Autodesk Inventor part; units mm, degrees
ref_plane "Work Plane1" through (0, 0, 400) normal (0, 0, 1) x (1, 0, 0)
ref_plane "Work Plane2" through (0, 0, 100) normal (0, 0, -1) x (-1, 0, 0)
ref_plane "YZ Plane" through (0, 0, 0) normal (1, 0, 0) x (0, 1, 0)
sketch "Sketch1" plane through (0, 0, 0) normal (0, 0, 1) x (1, 0, 0)
  line L0 (-7.5, 3.5) -> (7.5, 3.5)
  line L1 (7.5, 3.5) -> (7.5, -3.5)
  line L2 (7.5, -3.5) -> (-7.5, -3.5)
  line L3 (-7.5, -3.5) -> (-7.5, 3.5)
  line L4 (-7.5, 3.5) -> (7.5, -3.5) construction
  line L5 (7.5, 3.5) -> (-7.5, -3.5) construction
  line L6 (-12.5, 8.5) -> (12.5, 8.5)
  line L7 (12.5, 8.5) -> (12.5, -8.5)
  line L8 (12.5, -8.5) -> (-12.5, -8.5)
  line L9 (-12.5, -8.5) -> (-12.5, 8.5)
  line L10 (-12.5, 8.5) -> (12.5, -8.5) construction
  line L11 (12.5, 8.5) -> (-12.5, -8.5) construction
  line L12 (-7.5, 8.5) -> (-7.5, -8.5)
  point P0 (0, 0)
  dimension "d0" = 15
  dimension "d1" = 7
  dimension "d2" = 25
  dimension "d3" = 17
extrude "Extrusion1" add sketch "Sketch1" along normal blind 500 contours L12 L6 L7 L8 L2 L1 L0
ref_plane "Work Plane1" through (0, 0, 400) normal (0, 0, 1) x (1, 0, 0)
sketch "Sketch2" plane through (0, 0, 400) normal (0, 0, 1) x (1, 0, 0)
  line L0 (-27.5, 8.5) -> (52.5, 8.5)
  line L1 (52.5, 8.5) -> (52.5, -8.5)
  line L2 (52.5, -8.5) -> (-27.5, -8.5)
  line L3 (-27.5, -8.5) -> (-27.5, 8.5)
  line L4 (12.5, -8.5) -> (12.5, 8.5)
  line L5 (-27.5, 8.5) -> (52.5, -8.5) construction
  line L6 (52.5, 8.5) -> (-27.5, -8.5) construction
  line L7 (12.5, 0) -> (52.5, 0)
  line L8 (52.5, 0) -> (52.5, 8.5)
  line L9 (52.5, 8.5) -> (12.5, 8.5)
  line L10 (12.5, 8.5) -> (12.5, 0)
  point P0 (0, 0)
  point P1 (12.5, -6.5)
  point P2 (12.5, 6.5)
  point P3 (12.5, 6.5)
  dimension "d8" = 80
  dimension "d9" = 17
extrude "Extrusion2" add sketch "Sketch2" against normal blind 25 contours L0 L1 L7 L4
ref_plane "Work Plane2" through (0, 0, 100) normal (0, 0, -1) x (-1, 0, 0)
sketch "Sketch3" plane through (0, 0, 100) normal (0, 0, -1) x (-1, 0, 0)
  line L0 (-12.5, 8.5) -> (-12.5, 0)
  line L1 (-12.5, 8.5) -> (-52.5, 8.5)
  line L2 (-52.5, 8.5) -> (-52.5, 0)
  line L3 (-52.5, 0) -> (-12.5, 0)
  point P0 (0, 0)
extrude "Extrusion3" add sketch "Sketch3" against normal blind 25
fillet "Fillet2" radius 7 6 edges at (12.5, 4.25, 100) (12.5, 0, 112.5) (12.5, 4.25, 125) (12.5, 4.25, 375) (12.5, 0, 387.5) (12.5, 4.25, 400)
properties part number "GUIA DE TAPA PRINCIPAL"
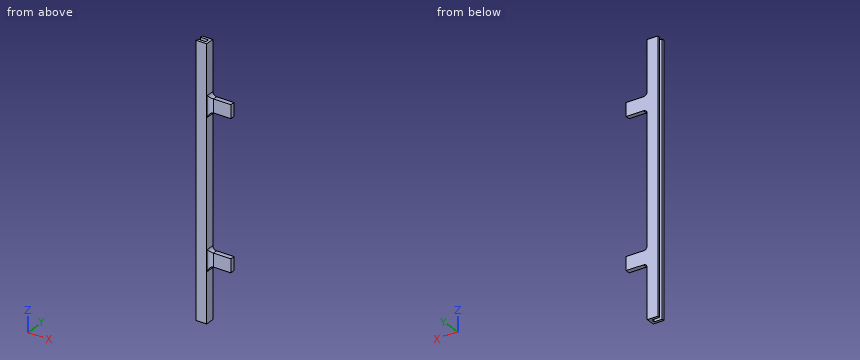
Build history of the part. All positions in model axes, mm. Round coordinates to 2 decimals unless told otherwise and drop trailing zeros. Write each loop counter-clockwise with the first axis right and the second up, starting at its lowest first coordinate (ties: lowest second). Pieces come first, ordered by that corner, then holes. Notation, with made-up numbers: (-32, -7) - (-8, -7) arc R13 ccw to (-8, 5) - close; hole circle Ø9 at (62, 64.25). An arc over 180 degrees is marked (long way). One line per question, with ' | ' between items.
1. Band-saw the part on A-A, the plane x = 1. Write the cut outline in (y, z), and give its area (3 significant figures).
Results are:
outline: (-8.5, 0) - (-3.5, 0) - (-3.5, 500) - (-8.5, 500) - close; (3.5, 0) - (8.5, 0) - (8.5, 500) - (3.5, 500) - close | area: 5,000 mm^2
2. Band-saw the part on C-C, the plane x = 34. Write the cut outline in (y, z).
Results are:
outline: (0, 100) - (8.5, 100) - (8.5, 125) - (0, 125) - close; (0, 375) - (8.5, 375) - (8.5, 400) - (0, 400) - close
3. Drop flat-ended pins along their axis: pin 1 Ø12.5 at (x, z) = (42, 114.5) entering from -Y; pin 2 Ø3.5 at (y, z) = (-0.5, 275.5) entering from -X; pin 3 Ø7 at (x, y) = (33.5, 3) entering from -Z; pin 4 Ø2 at (x, y) = (46.5, -2.5) entering from -Z. Give the stop position or say it passes through.
Results are:
pin 1: y = 0 | pin 2: x = 7.5 | pin 3: z = 100 | pin 4: through
4. Drill centre lines: line 1 along Y through (x, z) = (-0.5, 72); line 2 along Z through (x, y) = (40, 3.25); line 3 along X through (y, z) = (7.25, 142.5). Where is each one in solid material? Low to high. Write a range as from..to.
Results are:
line 1: -8.5..-3.5, 3.5..8.5 | line 2: 100..125, 375..400 | line 3: -7.5..12.5
5. Band-saw the part on D-D, the plane z = 113.5. Write the cut outline in (x, y), and give its area (3 significant figures).
Results are:
outline: (-7.5, -8.5) - (12.5, -8.5) - (12.5, -7) arc R7 cw to (19.5, 0) - (52.5, 0) - (52.5, 8.5) - (-7.5, 8.5) - (-7.5, 3.5) - (7.5, 3.5) - (7.5, -3.5) - (-7.5, -3.5) - close | area: 586 mm^2
6. Band-saw the part on B-B, the plane z = 61. Write the cut outline in (x, y).
Results are:
outline: (-7.5, -8.5) - (12.5, -8.5) - (12.5, 8.5) - (-7.5, 8.5) - (-7.5, 3.5) - (7.5, 3.5) - (7.5, -3.5) - (-7.5, -3.5) - close
